```python
from build123d import *

# Parameters (mm, degrees)
SKETCH1_R           = 4
BOSS_EXTRUDE1_DEPTH = 21.5
CUT_EXTRUDE1_START  = -3
SKETCH2_W           = 2.50000008
SKETCH2_H           = 3.251715676
CUT_EXTRUDE1_DEPTH  = 15
FILLET2_R           = 1.5
FILLET3_R           = 1.5


with BuildPart() as part:
    # Sketch1 → Boss-Extrude1 (new body)
    with BuildSketch(Plane.XY):
        Circle(SKETCH1_R)
    extrude(amount=BOSS_EXTRUDE1_DEPTH)

    # Sketch2 → Cut-Extrude1 (cut)
    with BuildSketch(Plane.XY.offset(21.5).offset(CUT_EXTRUDE1_START)):
        with Locations((-4, 0)):
            Rectangle(SKETCH2_W, SKETCH2_H)
    extrude(amount=-CUT_EXTRUDE1_DEPTH, mode=Mode.SUBTRACT)

    # Fillet2
    fillet2_edges = [part.edges().sort_by_distance(p)[0] for p in [
        (-3.202333166, -1.625857838, 3.5),
        (-3.202333166, 1.625857838, 3.5),
    ]]
    fillet(fillet2_edges, radius=FILLET2_R)

    # Fillet3
    fillet3_edges = [part.edges().sort_by_distance(p)[0] for p in [
        (-3.202333166, 1.625857838, 18.5),
        (-3.202333166, -1.625857838, 18.5),
    ]]
    fillet(fillet3_edges, radius=FILLET3_R)


solid = part.part
```
Design review of the part built by this model. Coordinates are the model's own, in mm. A direction names the side the tool comes from. Give positions to 0.01 mm unless a question says otherwise; leave off trailing zeros. Loops run counter-clockwise (first coordinate to the right, second up) from the corner with the lowest first, then second, coordinate; pieces in that order, holes last. Notation, with made-up numbers: (-35.75, 77) -> (13.25, 77) arc R30 cw to (13.25, 112) -> close; hole circle Ø9 at (20, 55). An arc over 180 degrees is marked (long way). Write each question's results on one line, items separated by ' | '.
Q1. Take a section at B-B, the plane z = 6.25. Write out the cut boundary in (x, y), plus the area to 3 significant figures.
Reply:
outline: (-3.65, -1.63) arc R4 ccw (long way) to (-3.65, 1.63) -> (-2.75, 1.63) -> (-2.75, -1.63) -> close | area: 46.6 mm²
Q2. For pin 1 Ø1 at (x, y) = (-0.5, 0.5) entering from -Z; pin 2 Ø3 at (y, z) = (0.5, 14) entering from -X; pin 3 Ø0.7 at (x, z) = (-3, 13) entering from -Y; pin 4 Ø1 at (x, z) = (-3.5, 10.5) entering from +Y, all flat-tipped, find the tip position at first contact; note any pin that passes through.
Reply:
pin 1: stops at z = 0 | pin 2: stops at x = -3.65 | pin 3: stops at y = -3 | pin 4: stops at y = 2.65
Q3. Wall thickness on L1, parallel to Y at x = -3.25, z = 10.5; L2, parallel to Y at x = -1.5, z = 14.25; L3, parallel to Y at x = -1.25, z = 17.5: over which ranges is each line inside the solid? List them lowest first.
Reply:
L1: y = -2.33 to -1.63, 1.63 to 2.33 | L2: y = -3.71 to 3.71 | L3: y = -3.8 to 3.8
Q4. Take a section at C-C, the plane x = -1. Write out the cut boundary in (y, z).
Reply:
outline: (-3.87, 0) -> (3.87, 0) -> (3.87, 21.5) -> (-3.87, 21.5) -> close
Q5. The part is to be moulded in two halves that separate along Y. For faces 3 (the face through (-3.227, -1.198, 18.049)), 4 (the face through (3.695, -1.532, 10.599)), 5 (the face through (-3.227, 1.175, 3.928)), 6 (the face through (0, 0, 21.5)), say which applies: +Y half, -Y half, draft (parallel to the pull), parting line (faces both ways), or undercut.
Reply:
face 3: undercut | face 4: parting line | face 5: undercut | face 6: draft
Q6. Machinability: for faces 1 (the face through (-3, -1.626, 11)), 2 (the face through (0, 0, 0)), which of the approach directions +Z, -Z, +X, -X, +Y, -Y give a long, thin tool a straight path to every point of the face, cutting with its end or side? Answer none if there is none.
Reply:
face 1: -X | face 2: -Z, +X, -X, +Y, -Y
Q7. Take a section at A-A, the plane y = 0.5. Write out the cut boundary in (x, z), plus the area to 3 significant figures.
Reply:
outline: (-3.97, 0) -> (3.97, 0) -> (3.97, 21.5) -> (-3.97, 21.5) -> (-3.97, 18.45) -> (-2.75, 18.45) -> (-2.75, 3.55) -> (-3.97, 3.55) -> close | area: 152 mm²
Q8. Take a section at D-D, the plane y = -1. Write out the cut boundary in (x, z).
Reply:
outline: (-3.87, 0) -> (3.87, 0) -> (3.87, 21.5) -> (-3.87, 21.5) -> (-3.87, 18.22) -> (-2.75, 18.22) -> (-2.75, 3.78) -> (-3.87, 3.78) -> close
